Check sheet for the modelled part. Datum: model origin and axes. Units: mm. Face numbers are marked on the shaded views. A direction names the side the tool comes from. Round coordinates to 2 decimals unless told otherwise and drop trailing zeros. Loops run counter-clockwise (first coordinate to the right, second up) from the corner with the lowest first, then second, coordinate; pieces in that order, holes last. Notation, with made-up numbers: (-28, 28) - (-4, 28) arc R19 cw to (-4, 41) - close; hole circle Ø5 at (-15.5, 12). An arc over 180 degrees is marked (long way). Return JSON: item names as keys, results as strings.
from build123d import *

# Parameters (mm, degrees)
F0_R     = 75.5
F1_DEPTH = 128
F3_DEPTH = 50


with BuildPart() as f1:
    # F0 (on Right) → F1 (new body)
    with BuildSketch(Plane.YZ):
        Circle(F0_R)
    extrude(amount=F1_DEPTH)

    # F2 (on face) → F3 (cut)
    with BuildSketch(Plane.YZ.offset(128)):
        with BuildLine():
            Line((-75.5, 0), (-37.75, 65.384918))
            ThreePointArc((-37.75, 65.384918), (-65.384918, 37.75), (-75.5, 0))
        make_face()
        with BuildLine():
            ThreePointArc((37.75, 65.384918), (0, 75.5), (-37.75, 65.384918))
            Line((-37.75, 65.384918), (37.75, 65.384918))
        make_face()
        with BuildLine():
            ThreePointArc((75.5, 0), (65.384918, 37.75), (37.75, 65.384918))
            Line((37.75, 65.384918), (75.5, 0))
        make_face()
        with BuildLine():
            ThreePointArc((37.75, -65.384918), (65.384918, -37.75), (75.5, 0))
            Line((75.5, 0), (37.75, -65.384918))
        make_face()
        with BuildLine():
            Line((37.75, -65.384918), (-37.75, -65.384918))
            ThreePointArc((-37.75, -65.384918), (0, -75.5), (37.75, -65.384918))
        make_face()
        with BuildLine():
            Line((-37.75, -65.384918), (-75.5, 0))
            ThreePointArc((-75.5, 0), (-65.384918, -37.75), (-37.75, -65.384918))
        make_face()
    extrude(amount=-F3_DEPTH, mode=Mode.SUBTRACT)


with BuildPart() as f1_1:
    # F4: moved
    add(f1.part)


solid = f1_1.part
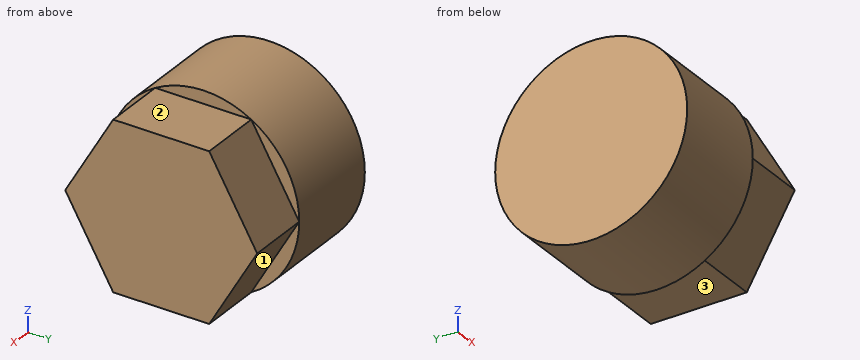
Q1. Depth check by flat-ended pin: P1, Ø5, axis at y = 1, z = -72, coming from the +X side; P2, Ø3, axis at x = 100, z = 33, coming from the -Y side; P3, Ø6, axis at x = 87.5, z = -24.5, coming from the +Y side. Enter the tip coordinate at first touch or a pass-through.
Answer key:
{"P1": "stops at x = 78", "P2": "stops at y = -57.31", "P3": "stops at y = 63.09"}
Q2. Sectioned sample at A-A (z = -32.5). Enter the section's corners in (x, y), plus the area to 3 significant figures.
Answer key:
{"outline": "(0, -68.15) - (78, -68.15) - (78, -56.74) - (128, -56.74) - (128, 56.74) - (78, 56.74) - (78, 68.15) - (0, 68.15) - close", "area": "16,300 mm²"}
Q3. Tool access check on the marked faces 1, 2 and 3. Record the directions out of +Z, -Z, +X, -X, +Y, -Y that give a thin tool (end or side, any length) a straight path to the whole face; none if there is none.
Answer key:
{"face 1": "-Z, +X, +Y", "face 2": "+Z, +X, +Y, -Y", "face 3": "-Z, +X, +Y, -Y"}
Q4. Sectioned sample at C-C (x = 24.5). Enter the section's corners in (y, z).
Answer key:
{"outline": "circle Ø151 at (0, 0)"}
Q5. Scan lines: probe 1 along Z at (x, y) = (117, 19); probe 2 along X at (y, z) = (-43, -59); probe 3 along Y at (x, z) = (33, -1). Record each from-to range of solid material in increasing order. Write a range as [from, to].
Answer key:
{"probe 1": "z = [-65.38, 65.38]", "probe 2": "x = [0, 78]", "probe 3": "y = [-75.49, 75.49]"}
Q6. Sectioned sample at B-B (y = 0). Enter the section's corners in (x, z).
Answer key:
{"outline": "(0, -75.5) - (78, -75.5) - (78, -65.38) - (128, -65.38) - (128, 65.38) - (78, 65.38) - (78, 75.5) - (0, 75.5) - close"}
